```python
from build123d import *

# Parameters (mm, degrees)
SKETCH1_W                 = 124
SKETCH1_H                 = 134
BOSS_EXTRUDE1_DEPTH       = 80
BOSS_EXTRUDE2_DEPTH       = 2
CUT_EXTRUDE3_DEPTH        = 80
FILLET1_R                 = 2
SKETCH5_R                 = 4
BOSS_EXTRUDE4_DEPTH       = 4
SKETCH9_R                 = 4
BOSS_EXTRUDE5_DEPTH       = 4
SKETCH10_R                = 3
CUT_EXTRUDE5_DEPTH        = 1
CUT_EXTRUDE5_DEPTH_BACK   = 135
FILLET3_R                 = 1
F_2_0MM_DOWEL_HOLE1_D     = 2
F_2_0MM_DOWEL_HOLE1_DEPTH = 20
F_2_0MM_DOWEL_HOLE1_TIP   = 0.600860619
SKETCH14_W                = 120
SKETCH14_H                = 1
BOSS_EXTRUDE6_DEPTH       = 40


with BuildPart() as part:
    # Sketch1 → Boss-Extrude1 (new body)
    with BuildSketch(Plane(origin=(0, 0, 0), x_dir=(1, 0, 0), z_dir=(0, 1, 0))):
        Rectangle(SKETCH1_W, SKETCH1_H)
    extrude(amount=BOSS_EXTRUDE1_DEPTH)

    # Sketch2 → Boss-Extrude2 (add)
    with BuildSketch(Plane(origin=(0, 80, 0), x_dir=(1, 0, 0), z_dir=(0, 1, 0))):
        with BuildLine():
            Line((57, 66), (-57, 66))
            ThreePointArc((-57, 66), (-58.171572875, 63.171572875), (-61, 62))
            Line((-61, 62), (-61, -62))
            ThreePointArc((-61, -62), (-58.171572875, -63.171572875), (-57, -66))
            Line((-57, -66), (57, -66))
            ThreePointArc((57, -66), (58.171572875, -63.171572875), (61, -62))
            Line((61, -62), (61, 62))
            ThreePointArc((61, 62), (58.171572875, 63.171572875), (57, 66))
        make_face()
    extrude(amount=BOSS_EXTRUDE2_DEPTH)

    # Sketch3 → Cut-Extrude3 (cut)
    with BuildSketch(Plane(origin=(0, 82, 0), x_dir=(1, 0, 0), z_dir=(0, 1, 0))):
        with BuildLine():
            Line((56.101020514, 65), (-56.101020514, 65))
            ThreePointArc((-56.101020514, 65), (-57.464466094, 62.464466094), (-60, 61.101020514))
            Line((-60, 61.101020514), (-60, -61.101020514))
            ThreePointArc((-60, -61.101020514), (-57.464466094, -62.464466094), (-56.101020514, -65))
            Line((-56.101020514, -65), (56.101020514, -65))
            ThreePointArc((56.101020514, -65), (57.464466094, -62.464466094), (60, -61.101020514))
            Line((60, -61.101020514), (60, 61.101020514))
            ThreePointArc((60, 61.101020514), (57.464466094, 62.464466094), (56.101020514, 65))
        make_face()
    extrude(amount=-CUT_EXTRUDE3_DEPTH, mode=Mode.SUBTRACT)

    # Fillet1
    fillet1_edges = [part.edges().sort_by_distance(p)[0] for p in [
        (0, 0, -67),
        (62, 0, 0),
        (0, 0, 67),
        (-62, 0, 0),
        (-62, 40, -67),
        (62, 40, -67),
        (62, 40, 67),
        (-62, 40, 67),
    ]]
    fillet(fillet1_edges, radius=FILLET1_R)

    # Sketch5 → Boss-Extrude4 (add)
    with BuildSketch(Plane.XY.offset(67)):
        with Locations((0, 10)):
            Circle(SKETCH5_R)
    extrude(amount=-BOSS_EXTRUDE4_DEPTH)

    # Sketch9 → Boss-Extrude5 (add)
    with BuildSketch(Plane(origin=(0, 0, -67), x_dir=(-1, 0, 0), z_dir=(0, 0, -1))):
        with Locations((0, 10)):
            Circle(SKETCH9_R)
    extrude(amount=-BOSS_EXTRUDE5_DEPTH)

    # Sketch10 → Cut-Extrude5 (cut, two sides)
    with BuildSketch(Plane(origin=(0, 0, -67), x_dir=(-1, 0, 0), z_dir=(0, 0, -1))) as cut_extrude5_sk:
        with Locations((0, 10)):
            Circle(SKETCH10_R)
    extrude(amount=CUT_EXTRUDE5_DEPTH, mode=Mode.SUBTRACT)
    extrude(cut_extrude5_sk.sketch, amount=-CUT_EXTRUDE5_DEPTH_BACK, mode=Mode.SUBTRACT)

    # Fillet3
    fillet3_edges = [part.edges().sort_by_distance(p)[0] for p in [
        (3, 10, -67),
        (3, 10, 67),
    ]]
    fillet(fillet3_edges, radius=FILLET3_R)

    # Ø2.0mm Dowel Hole1
    with Locations(Plane(origin=(59.5, 80, -64.5), x_dir=(0, 0, 1), z_dir=(0, 1, 0))):
        with Locations((0, 0), (129, 0), (129, -119), (0, -119)):
            Hole(F_2_0MM_DOWEL_HOLE1_D / 2, depth=F_2_0MM_DOWEL_HOLE1_DEPTH)
            with Locations((0, 0, -(F_2_0MM_DOWEL_HOLE1_DEPTH + F_2_0MM_DOWEL_HOLE1_TIP / 2))):  # 118° drill point
                Cone(0, F_2_0MM_DOWEL_HOLE1_D / 2, F_2_0MM_DOWEL_HOLE1_TIP, mode=Mode.SUBTRACT)

    # Sketch14 → Boss-Extrude6 (add)
    with BuildSketch(Plane(origin=(0, 2, 0), x_dir=(1, 0, 0), z_dir=(0, 1, 0))):
        with Locations((0, 6.5)):
            Rectangle(SKETCH14_W, SKETCH14_H)
    extrude(amount=BOSS_EXTRUDE6_DEPTH)


solid = part.part
```
Geometry: final body of the model. Coordinates: model frame, mm. A direction names the side the tool comes from. Coordinates: 2 decimals unless noted, no trailing zeros. Order: outer loops, then holes, each group sorted by start corner. A loop starts at its lowest first (then second) coordinate and runs counter-clockwise, first axis right, second up. Notation, with made-up numbers: (43, 71) - (80, 71) arc R24 ccw to (80, 102) - close; hole circle Ø9 at (-30, 77). An arc over 180 degrees is marked (long way). Write each question's results on one line, items separated by ' | '.
1) Section D-D, the plane z = -11.5. Return loops of the section in (x, y).
Results list:
outline: (-62, 2) arc R2 ccw to (-60, 0) - (60, 0) arc R2 ccw to (62, 2) - (62, 80) - (61, 80) - (61, 82) - (60, 82) - (60, 2) - (-60, 2) - (-60, 82) - (-61, 82) - (-61, 80) - (-62, 80) - close
2) Section B-B, the plane x = 0. State how many separate pieces and enclosed holes the cut face has, plus the area to 3 significant figures.
Results list:
separate pieces: 3 | enclosed holes: 0 | area: 605 mm^2
3) Pull-direction query (Y, two-part tool) for faces 6 (the flat face through (-1, 13, -63)), 7 (the cylindrical face through (3, 10, -65)), 8 (the flat face through (-1, 0, -1)); classes: pulls with the +Y half, pulls with the -Y half, needs draft (parallel to the pull), parting line crosses it, or undercut.
Results list:
face 6: needs draft | face 7: undercut | face 8: pulls with the -Y half
4) Section A-A, the plane y = 53.5. Return loops of the section in (x, z), plus the area to 3 significant figures.
Results list:
outline: (-62, -65) arc R2 ccw to (-60, -67) - (60, -67) arc R2 ccw to (62, -65) - (62, 65) arc R2 ccw to (60, 67) - (-60, 67) arc R2 ccw to (-62, 65) - close; hole (-60, -61.1) arc R5 cw to (-56.1, -65) - (56.1, -65) arc R5 cw to (60, -61.1) - (60, 61.1) arc R5 cw to (56.1, 65) - (-56.1, 65) arc R5 cw to (-60, 61.1) - close | area: 1,060 mm^2
5) Pin query (flat end, axial travel): pin 1 (0.6 mm diameter, centred on y = 81, z = -3, fed in from +X); pin 2 (0.8 mm diameter, centred on x = 27, z = -6.5, fed in from +Y); pin 3 (2.5 mm diameter, centred on x = 0.5, y = 10, fed in from +Z). Return the tip coordinate at first contact, or that it passes through.
Results list:
pin 1: x = 61 | pin 2: y = 42 | pin 3: z = -6
6) Line query: line 1 (Z direction, x = 50, y = 40.5); line 2 (Y direction, x = 0, z = -63.8); line 3 (X direction, y = 12.5, z = 4.5). Output: solid intervals per line, ascending. Write a range as from..to.
Results list:
line 1: -67..-65, -7..-6, 65..67 | line 2: 0..2, 6..7, 13..14 | line 3: -62..-60, 60..62
7) Set-up query: faces 1 (the cylindrical face through (-58.203, 80.986, 63.141)), 2 (the cylindrical face through (0.521, 13.966, -64.014)), 3 (the cylindrical face through (58.203, 80.986, -63.141)), 4 (the cylindrical face through (-58.141, 80.986, -63.203)), 5 (the cylindrical face through (57.44, 42.56, 62.49)). Return all of +Z, -Z, +X, -X, +Y, -Y with unobstructed straight access to the full face (end or side cutting, diameter ignored); none if empty.
Results list:
face 1: +Z, -X, +Y | face 2: none | face 3: -Z, +X, +Y | face 4: -Z, -X, +Y | face 5: +Y
8) Section C-C, the plane y = 16. Return loops of the section in (x, z).
Results list:
outline: (-62, -65) arc R2 ccw to (-60, -67) - (60, -67) arc R2 ccw to (62, -65) - (62, 65) arc R2 ccw to (60, 67) - (-60, 67) arc R2 ccw to (-62, 65) - close; hole (-60, -61.1) arc R5 cw to (-56.1, -65) - (56.1, -65) arc R5 cw to (60, -61.1) - (60, -7) - (-60, -7) - close; hole (-60, -6) - (60, -6) - (60, 61.1) arc R5 cw to (56.1, 65) - (-56.1, 65) arc R5 cw to (-60, 61.1) - close
